Input: part model. Units: mm. Frame: model coordinates. Face numbers are marked on the shaded views. A direction names the side the tool comes from. Give positions to 0.01 mm unless a question says otherwise; leave off trailing zeros. Order: outer loops, then holes, each group sorted by start corner. A loop starts at its lowest first (then second) coordinate and runs counter-clockwise, first axis right, second up. Notation, with made-up numbers: (-38.75, 11) - (-25.75, 11) arc R30 cw to (-25.75, 41) - close; hole circle Ø6 at (-28.75, -1). An arc over 180 degrees is marked (long way). Use a Markdown table: item, result.
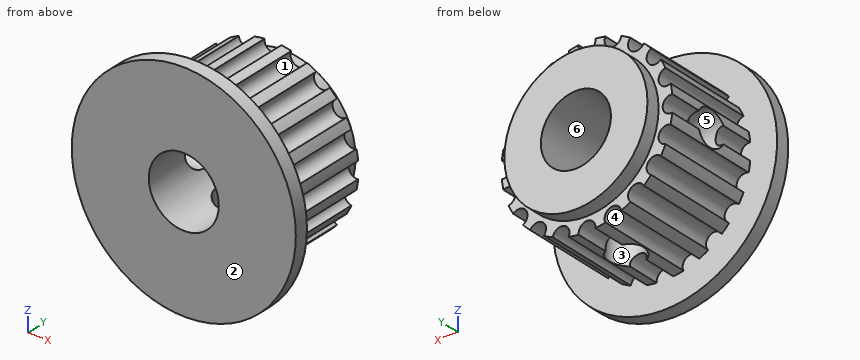
Autodesk Inventor part; units mm, degrees
ref_plane "YZ Plane" through (0, 0, 0) normal (1, 0, 0) x (0, 1, 0)
ref_plane "XZ Plane" through (0, 0, 0) normal (0, 1, 0) x (-1, 0, 0)
ref_plane "XY Plane" through (0, 0, 0) normal (0, 0, 1) x (1, 0, 0)
sketch "Sketch1" plane through (0, 0, 0) normal (0, 0, 1) x (1, 0, 0)
  line L0 (0, 0) -> (2.5, 0) construction
  line L1 (8, 0) -> (8, 1)
  line L2 (8, 1) -> (6.11, 1)
  line L3 (6.11, 1) -> (6.11, 8)
  line L4 (6.11, 8) -> (5.11, 8)
  line L5 (5.11, 8) -> (5.11, 9)
  line L6 (5.11, 9) -> (2.5, 9)
  line L7 (0, 9) -> (0, 0) construction
  line L8 (2.5, 9) -> (2.5, 0)
  line L9 (2.5, 9) -> (0, 9) construction
  line L10 (2.5, 0) -> (8, 0)
  dimension "d0" = 7
  dimension "d1" = 1
  dimension "d2" = 8
  dimension "d3" = 6.11
  dimension "d5" = 1
  dimension "d6" = 1
  dimension "d15" = 2.5
revolve "Revolution1" add sketch "Sketch1" angle 360 about axis through (0, 9, 0) along (0, -1, 0)
sketch "Sketch2" plane through (0, 8, 0) normal (0, 1, 0) x (1, 0, 0)
  circle A0 centre (0, 0) radius 5.11 construction
  line L0 (0, 0) -> (-6, 0) construction
  circle A1 centre (-6, 0) radius 0.6
  point P0 (0, 0)
  dimension "d8" = 1.2
  dimension "d9" = 6
extrude "Extrusion1" cut sketch "Sketch2" against normal up to surface (7 mm away)
pattern_circular "Circular Pattern1" count 20 over 360 about axis through (0, 8.5, 0) along (0, -1, 0) of "Extrusion1"
sketch "Sketch3" plane through (0, 0, 0) normal (1, 0, 0) x (0, 1, 0)
  line L0 (1, 8) -> (1, -8) construction
  line L1 (8, 0) -> (1, 0) construction
  circle A0 centre (4.5, 0) radius 1.25
  line L2 (8, 5.11) -> (8, -5.11) construction
  dimension "d16" = 2.5
extrude "Extrusion2" cut sketch "Sketch3" against normal blind 10
pattern_circular "Circular Pattern2" count 2 over 90 about axis through (0, 4.5, 0) along (0, -1, 0) of "Extrusion2"
properties part number "GT2Pulley_20T_5mm_noTop"
1. Section query B-B (z = 0). Return loops of the section in (x, y).
Response:
| item | result |
|---|---|
| outline | (-8, 0) - (-2.5, 0) - (-2.5, 3.25) - (-5.4, 3.25) - (-5.4, 1) - (-8, 1) - close; (-5.4, 5.75) - (-2.5, 5.75) - (-2.5, 9) - (-5.11, 9) - (-5.11, 8) - (-5.4, 8) - close; (2.5, 0) - (8, 0) - (8, 1) - (5.4, 1) - (5.4, 8) - (5.11, 8) - (5.11, 9) - (2.5, 9) - close |
2. Mould query, pull axis Y, two halves, no side actions, for the marked faces 1, 2 and 3. Classes: pulls with the +Y half, pulls with the -Y half, needs draft (parallel to the pull), parting line crosses it, or undercut.
Response:
| item | result |
|---|---|
| face 1 | needs draft |
| face 2 | pulls with the -Y half |
| face 3 | undercut |
3. Section query D-D (x = 3.5). Return loops of the section in (y, z).
Response:
| item | result |
|---|---|
| outline | (0, -7.19) - (1, -7.19) - (1, -4.25) - (8, -4.25) - (8, -3.72) - (9, -3.72) - (9, 3.72) - (8, 3.72) - (8, 4.25) - (1, 4.25) - (1, 7.19) - (0, 7.19) - close |
4. Pin query (flat end, axial travel): pin 1 (2 mm diameter, centred on y = 5, z = -4.5, fed in from -X); pin 2 (3 mm diameter, centred on x = 0, y = 4.5, fed in from +Z); pin 3 (1.4 mm diameter, centred on x = -5.71, z = 1.85, fed in from +Y). Return the tip coordinate at first contact, or that it passes through.
Response:
| item | result |
|---|---|
| pin 1 | stops at x = -4.57 |
| pin 2 | stops at z = 6.08 |
| pin 3 | stops at y = 8 |
5. Section query A-A (x = 0). Return loops of the section in (y, z).
Response:
| item | result |
|---|---|
| outline | (0, -8) - (1, -8) - (1, -5.4) - (3.25, -5.4) - (3.25, -2.5) - (0, -2.5) - close; (0, 2.5) - (9, 2.5) - (9, 5.11) - (8, 5.11) - (8, 5.4) - (1, 5.4) - (1, 8) - (0, 8) - close; (5.75, -5.4) - (8, -5.4) - (8, -5.11) - (9, -5.11) - (9, -2.5) - (5.75, -2.5) - close |
6. Section query C-C (x = -3.5). Return loops of the section in (y, z), then the cut area to 3 significant figures.
Response:
| item | result |
|---|---|
| outline | (0, -7.19) - (1, -7.19) - (1, -4.25) - (8, -4.25) - (8, -3.72) - (9, -3.72) - (9, 3.72) - (8, 3.72) - (8, 4.25) - (1, 4.25) - (1, 7.19) - (0, 7.19) - close; hole circle Ø2.5 at (4.5, 0) |
| area | 76.5 mm^2 |
7. Material intervals for line 1 along Z through (x, y) = (0, 6.5); line 2 along Z through (x, y) = (3, 3.25); line 3 along Y through (x, z) = (5.25, -5.25), sorted ascending.
Response:
| item | result |
|---|---|
| line 1 | z = -5.4 to -2.5, 2.5 to 5.4 |
| line 2 | z = -5.32 to -5.14, -4.57 to 4.57, 5.14 to 5.32 |
| line 3 | y = 0 to 1 |
8. Set-up query: the marked faces 4, 5 and 6. Return all of +Z, -Z, +X, -X, +Y, -Y with unobstructed straight access to the full face (end or side cutting, diameter ignored); none if empty.
Response:
| item | result |
|---|---|
| face 4 | +Y |
| face 5 | -X |
| face 6 | +Y, -Y |
